Autodesk Inventor part; units mm, degrees
ref_plane "YZ Plane" through (0, 0, 0) normal (1, 0, 0) x (0, 1, 0)
ref_plane "XZ Plane" through (0, 0, 0) normal (0, 1, 0) x (-1, 0, 0)
ref_plane "XY Plane" through (0, 0, 0) normal (0, 0, 1) x (1, 0, 0)
sketch "Szkic1" plane through (0, 0, 0) normal (0, 1, 0) x (-1, 0, 0)
  line L0 (0, 0) -> (40, 0)
  line L1 (40, 0) -> (40, 20)
  line L2 (40, 20) -> (0, 20)
  line L3 (0, 20) -> (0, 0)
  dimension "d0" = 40
  dimension "d1" = 20
extrude "Wyciągnięcie proste1" add sketch "Szkic1" along normal blind 12
sketch "Szkic2" plane through (0, 12, 0) normal (0, 1, 0) x (1, 0, 0)
  point P0 (0, 0)
sketch "Szkic3" plane through (0, 0, 20) normal (1, 0, 0) x (0, 0, -1)
  line L0 (0, 0) -> (0, 12)
  line L1 (0, 6) -> (6.75, 6)
  circle A0 centre (6.75, 6) radius 4.75
  point P0 (20, 0)
  dimension "d4" = 6.75
  dimension "d5" = 9.5
extrude "Wyciągnięcie proste2" add sketch "Szkic3" along normal blind 2.5
sketch "Szkic4" plane through (2.5, 6, 13.25) normal (1, 0, 0) x (0, 0, -1)
  circle A0 centre (0, 0) radius 3.85
  point P0 (13.25, -6)
  dimension "d8" = 7.7
extrude "Wyciągnięcie proste3" add sketch "Szkic4" along normal blind 6
sketch "Szkic5" plane through (8.5, 6, 13.25) normal (1, 0, 0) x (0, 0, -1)
  circle A0 centre (0, 0) radius 4.75
  point P0 (13.25, -6)
extrude "Wyciągnięcie proste4" add sketch "Szkic5" along normal blind 8 draft -10
mirror "Odbij1" about plane through (0, 0, 0) normal (0, 0, 1) of "Wyciągnięcie proste4", "Wyciągnięcie proste3", "Wyciągnięcie proste2", "Wyciągnięcie proste1"
properties part number "blokwodny" material "Żywica fenolowa"
The listing builds one solid part. Answer for the finished solid, in the listing's coordinates (mm). A direction names the side the tool comes from. Give positions to 0.01 mm unless a question says otherwise; leave off trailing zeros. Loops run counter-clockwise (first coordinate to the right, second up) from the corner with the lowest first, then second, coordinate; pieces in that order, holes last. Notation, with made-up numbers: (-27.5, -9) - (-12.5, -9) arc R22 cw to (-12.5, 15) - close; hole circle Ø2 at (-32, 76). An arc over 180 degrees is marked (long way). Answer as a JSON object with one key per item and string values.
1. A cutting plane is placed at B-B (z = -13.25). Write down the section's boundary in (x, y), then the cut area to 3 significant figures.
Determined:
{"outline": "(-40, 0) - (0, 0) - (0, 1.25) - (2.5, 1.25) - (2.5, 2.15) - (8.5, 2.15) - (8.5, 1.25) - (16.5, 2.66) - (16.5, 9.34) - (8.5, 10.75) - (8.5, 9.85) - (2.5, 9.85) - (2.5, 10.75) - (0, 10.75) - (0, 12) - (-40, 12) - close", "area": "615 mm²"}
2. Find the intervals of material crossed by L1, parallel to X at y = 10.75, z = 4; L2, parallel to Y at x = 1, z = -13; L3, parallel to Z at x = 0.5, y = 3, in increasing order. Write a range as [from, to].
Determined:
{"L1": "[-40, 0]", "L2": "[1.26, 10.74]", "L3": "[-16.93, -9.57], [9.57, 16.93]"}
3. A cutting plane is placed at C-C (z = -4). Write down the section's boundary in (x, y), then the cut area to 3 significant figures.
Determined:
{"outline": "(-40, 0) - (0, 0) - (0, 12) - (-40, 12) - close", "area": "480 mm²"}
4. For faces 1 (the cylindrical face through (5.458, 5.831, 17.096)), 2 (the flat face through (-20, 0, 0)), 3 (the flat face through (0, 6, 0)), determine the directions among +Z, -Z, +X, -X, +Y, -Y from which every point of the face is accessible in a straight line to the end or side of a thin tool.
Determined:
{"face 1": "none", "face 2": "+Z, -Z, +X, -X, -Y", "face 3": "+X"}
5. A cutting plane is placed at A-A (y = 6). Write down the section's boundary in (x, z).
Determined:
{"outline": "(-40, -20) - (0, -20) - (0, -18) - (2.5, -18) - (2.5, -17.1) - (8.5, -17.1) - (8.5, -18) - (16.5, -16.59) - (16.5, -9.91) - (8.5, -8.5) - (8.5, -9.4) - (2.5, -9.4) - (2.5, -8.5) - (0, -8.5) - (0, 8.5) - (2.5, 8.5) - (2.5, 9.4) - (8.5, 9.4) - (8.5, 8.5) - (16.5, 9.91) - (16.5, 16.59) - (8.5, 18) - (8.5, 17.1) - (2.5, 17.1) - (2.5, 18) - (0, 18) - (0, 20) - (-40, 20) - close"}
6. For a pull along Z with two mould halves and no side action, classify faces 4 (the flat face through (-20, 6, 20)), 5 (the cylindrical face through (1.23, 7.43, -8.72)), 6 (the flat face through (-20, 6, -20)), 7 (the flat face through (-40, 6, 0)) as pulls with the +Z half, pulls with the -Z half, needs draft (parallel to the pull), parting line crosses it, or undercut.
Determined:
{"face 4": "pulls with the +Z half", "face 5": "undercut", "face 6": "pulls with the -Z half", "face 7": "needs draft"}
7. A flat-ended cylindrical pin translates along its axis: pin 1 Ø5 at (x, z) = (8.5, -6.5) entering from +Y. Find the tip coordinate at first contact, or state that the pin passes through.
Determined:
{"pin 1": "y = 8.12"}
